Autodesk Inventor part; units mm, degrees
ref_plane "Work Plane1" through (0, 0, -15) normal (0, 0, 1) x (1, 0, 0)
ref_plane "YZ Plane" through (0, 0, 0) normal (1, 0, 0) x (0, 1, 0)
ref_plane "XZ Plane" through (0, 0, 0) normal (0, 1, 0) x (-1, 0, 0)
sketch "Sketch1" plane through (0, 0, 0) normal (0, 0, 1) x (1, 0, 0)
  line L0 (0, 0) -> (25, 0)
  line L1 (25, 0) -> (25, 40)
  line L2 (25, 40) -> (0, 40)
  line L3 (0, 40) -> (0, 0)
  dimension "d1" = 25
  dimension "d2" = 40
  dimension "d3" = 25
extrude "Extrusion1" add sketch "Sketch1" against normal blind 30
sketch "Sketch2" plane through (25, 0, 0) normal (1, 0, 0) x (0, 0, -1)
  line L0 (0, 0) -> (30, 0)
  circle A0 centre (15, 6.56) radius 2.46
extrude "Extrusion2" cut sketch "Sketch2" against normal blind 30
sketch "Sketch3" plane through (0, 0, 0) normal (-1, 0, 0) x (0, 0, 1)
  line L0 (0, 0) -> (-30, 0)
  line L1 (-25.05, 0) -> (-4.95, 0)
  line L2 (-4.95, 0) -> (-4.95, 33.12)
  line L3 (-4.95, 33.12) -> (-25.05, 33.12)
  line L4 (-25.05, 33.12) -> (-25.05, 0)
  dimension "d11" = 20.1
extrude "Extrusion3" cut sketch "Sketch3" against normal blind 20
sketch "Sketch4" plane through (0, 0, 0) normal (0, -1, 0) x (1, 0, 0)
  line L0 (20, -4.95) -> (20, -25.05)
  line L1 (20, -15) -> (25, -15)
  line L2 (25, 0) -> (25, -30)
  line L3 (20, -8.025) -> (25, -8.025)
  line L4 (25, -8.025) -> (25, -21.975)
  line L5 (25, -21.975) -> (20, -21.975)
  line L6 (20, -21.975) -> (20, -8.025)
  line L7 (20, -8.025) -> (25, -21.975) construction
  line L8 (25, -8.025) -> (20, -21.975) construction
  line L9 (25, -12.54) -> (25, -17.46)
  point P0 (0, 0)
  point P1 (22.5, -15)
  dimension "d14" = 13.95
extrude "Extrusion4" add sketch "Sketch4" along normal blind 15
sketch "Sketch5" plane through (20, 0, 0) normal (-1, 0, 0) x (0, 0, 1)
  circle A0 centre (-15, 6.56) radius 2.46
  circle A1 centre (-15, 6.56) radius 4.7025
  circle A2 centre (-15, 6.56) radius 2.46
  circle A3 centre (-15, 6.56) radius 2.46
  point P0 (0, 0)
  dimension "d17" = 9.405
extrude "Extrusion5" cut sketch "Sketch5" against normal blind 2.1
sketch "Sketch6" plane through (25, 0, 0) normal (1, 0, 0) x (0, 0, -1)
  circle A0 centre (15, 6.56) radius 4.7025
  line L0 (15, 6.56) -> (15, 23.56)
  circle A1 centre (15, 23.56) radius 2.46
  point P0 (0, 0)
  dimension "d20" = 17
  dimension "d21" = 4.92
extrude "Extrusion6" cut sketch "Sketch6" against normal blind 10 contours A1
sketch "Sketch7" plane through (20, 0, 0) normal (-1, 0, 0) x (0, 0, 1)
  circle A0 centre (-15, 23.56) radius 2.46
  circle A1 centre (-15, 23.56) radius 4.7025
  point P0 (0, 0)
  dimension "d24" = 9.405
extrude "Extrusion7" cut sketch "Sketch7" against normal blind 2.1
sketch "Sketch9" plane through (25, 0, 0) normal (1, 0, 0) x (0, 0, -1)
  circle A0 centre (15, 6.56) radius 2.46
  circle A1 centre (15, 6.56) radius 2.46
  circle A2 centre (15, 23.56) radius 2.46
  circle A3 centre (15, 23.56) radius 2.46
  line L0 (30, 40) -> (30, 0)
  line L1 (30, 0) -> (30, 40)
  line L2 (30, 40) -> (0, 40)
  line L3 (0, 40) -> (0, 0)
  line L4 (0, 0) -> (8.025, 0)
  line L5 (21.975, 0) -> (21.975, -15)
  line L6 (21.975, -15) -> (8.025, -15)
  line L7 (8.025, -15) -> (8.025, 0)
  line L8 (0, 0) -> (8.025, 0)
  line L9 (21.975, 0) -> (30, 0)
extrude "Extrusion8" add sketch "Sketch9" along normal blind 5
sketch "Sketch10" plane through (0, 40, 0) normal (0, 1, 0) x (1, 0, 0)
  line L0 (0, 30) -> (30, 30)
  line L1 (30, 0) -> (0, 0)
  line L2 (0, 30) -> (30, 30)
  line L3 (30, 30) -> (30, 0)
  line L4 (30, 0) -> (0, 0)
  line L5 (0, 0) -> (0, 30)
extrude "Extrusion9" add sketch "Sketch10" along normal blind 30
sketch "Sketch12" plane through (30, 0, 0) normal (1, 0, 0) x (0, 0, -1)
  circle A0 centre (15, 6.56) radius 2.46
  line L0 (15, 6.56) -> (15, 15.06)
  circle A1 centre (15, 15.06) radius 2.525
  point P0 (0, 0)
  dimension "d31" = 8.5
  dimension "d33" = 5.05
extrude "Extrusion10" cut sketch "Sketch12" against normal blind 30 contours A1
sketch "Sketch14" plane through (0, 0, 0) normal (0, 0, 1) x (1, 0, 0)
  line L0 (30, 70) -> (0, 70)
  line L1 (0, 100) -> (-8, 100)
  line L2 (30, 0) -> (30, 70)
  line L3 (30, 118) -> (30, 70)
  line L4 (30, 105) -> (30, 100)
  line L5 (0, 70) -> (30, 70)
  line L6 (0, 70) -> (0, 100)
  line L7 (30, 122.5) -> (30, 118)
  line L8 (-2, 150) -> (-8, 152)
  line L9 (-2, 102) -> (-8, 100)
  line L10 (-2, 102) -> (4, 126)
  line L11 (4, 126) -> (-2, 150)
  line L12 (-8, 152) -> (15, 152)
  line L13 (30, 137) -> (15, 152)
  line L14 (30, 122.5) -> (30, 137)
  point P0 (0, 0)
  dimension "d47" = 30
extrude "Extrusion12" add sketch "Sketch14" against normal blind 30
sketch "Sketch15" plane through (0, 0, -25.05) normal (-1, 0, 0) x (0, 0, 1)
  line L0 (0, 33.12) -> (20.1, 33.12)
  line L1 (20.1, 33.12) -> (20.1, 0)
  line L2 (0, 33.12) -> (20.1, 33.12)
  line L3 (20.1, 33.12) -> (20.1, 31.1)
  line L4 (20.1, 31.1) -> (0, 31.1)
  line L5 (0, 31.1) -> (0, 33.12)
  point P0 (25.05, 0)
  dimension "d57" = 2.02
extrude "Extrusion13" add sketch "Sketch15" against normal blind 20
sketch "Sketch25" plane through (0, 0, 0) normal (0, 0, 1) x (1, 0, 0)
  point P0 (0, 0)
sketch "Sketch26" plane through (0, 0, 0) normal (0, 0, 1) x (1, 0, 0)
  line L0 (-8, 100) -> (0, 100)
  line L1 (0, 100) -> (-8, 100)
  line L2 (-8, 100) -> (-2, 102)
  line L3 (-8, 100) -> (-2, 102)
  line L4 (-2, 102) -> (4, 126)
  line L5 (-2, 102) -> (4, 126)
  line L6 (4, 126) -> (-2, 150)
  line L7 (4, 126) -> (-2, 150)
  line L8 (-8, 152) -> (-2, 150)
  line L9 (-2, 150) -> (-8, 152)
  line L10 (15, 152) -> (-8, 152)
  line L11 (-8, 152) -> (15, 152)
  line L12 (30, 137) -> (15, 152)
  line L13 (15, 152) -> (30, 137)
  line L14 (30, 137) -> (30, 92)
  line L15 (30, 0) -> (30, 137)
  line L16 (30, 92) -> (0, 92)
  line L17 (0, 0) -> (0, 100)
  line L18 (0, 100) -> (0, 92)
  dimension "d93" = 45
extrude "Extrusion14" add sketch "Sketch26" along normal blind 45
ref_plane "Work Plane1" through (0, 0, -15) normal (0, 0, 1) x (1, 0, 0)
mirror "Mirror1" about plane through (0, 0, -15) normal (0, 0, 1) of "Extrusion14"
properties part number "48mm_x_120mm"
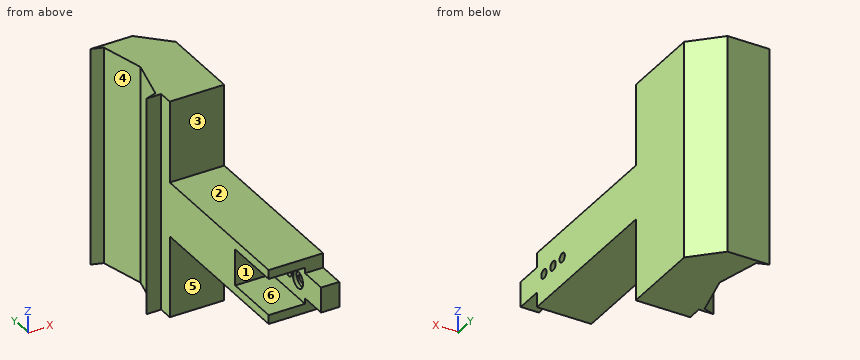
Geometry check sheet. Reference: the model listing, model coordinates, mm. Face numbers are marked on the shaded views. A direction names the side the tool comes from. Round coordinates to 2 decimals unless told otherwise and drop trailing zeros. Order: outer loops, then holes, each group sorted by start corner. A loop starts at its lowest first (then second) coordinate and runs counter-clockwise, first axis right, second up. Notation, with made-up numbers: (-1.75, 64) - (40.25, 64) arc R21 ccw to (40.25, 74) - close; hole circle Ø7 at (48.25, 84.25). An arc over 180 degrees is marked (long way). Use a Markdown table: item, result. Add a question column.
1) Thickness scan on line 1 along Z through (x, y) = (27.5, 23.56); line 2 along Z through (x, y) = (1.5, 25.5); line 3 along Y through (x, z) = (26.5, -15) (3 decimals). Record the ranges inside material, lowest first.
2) Section check A-A (z = -15). Count the separate pieces of the cut face and the enclosed holes in it, then the cut area to 3 significant figures.
3) Section check D-D (z = 24). Record the cut outline in (x, y), then the cut area to 3 significant figures.
4) Gauge pin test, flat ends, axial feed: P1, Ø9, axis at x = -6, z = -11, coming from the -Y side; P2, Ø12, axis at x = 2, z = -38.5, coming from the -Y side; P3, Ø4, axis at x = 22, z = -3, coming from the -Y side; P4, Ø3, axis at y = 6.56, z = -15, coming from the +X side. Record the tip position at first contact, or that the pin passes through.
5) Set-up check for the marked faces 4, 5 and 6: record each of +Z, -Z, +X, -X, +Y, -Y from which the full face is reachable in a straight line by a thin tool's end or side.
6) Section check C-C (y = 6.56). Record the cut outline in (x, z), then the cut area to 3 significant figures.
7) Section check B-B (x = 24). Record the cut outline in (y, z) (3 decimals), then the cut area to 3 significant figures.
8) Mould release check, pull along Z, two halves, no side actions. Record for the marked faces 1, 2 and 3: released by +Z, released by -Z, zero draft, split by the parting line, or undercut.
Established:
| question | item | result |
|---|---|---|
| 1 | line 1 | -30 to -17.46, -12.54 to 0 |
| 1 | line 2 | -30 to -25.05, -4.95 to 0 |
| 1 | line 3 | -15 to 4.1, 9.02 to 12.535, 17.585 to 21.1, 26.02 to 140.5 |
| 2 | separate pieces | 4 |
| 2 | enclosed holes | 0 |
| 2 | area | 3,780 mm2 |
| 3 | outline | (-8, 100) - (0, 100) - (0, 92) - (30, 92) - (30, 137) - (15, 152) - (-8, 152) - (-2, 150) - (4, 126) - (-2, 102) - close |
| 3 | area | 1,660 mm2 |
| 4 | P1 | y = 100 |
| 4 | P2 | y = 92 |
| 4 | P3 | y = 0 |
| 4 | P4 | through |
| 5 | face 4 | +Z, -Z, -X |
| 5 | face 5 | -Z, +X, -X, -Y |
| 5 | face 6 | -X, -Y |
| 6 | outline | (0, -30) - (30, -30) - (30, -17.46) - (22.1, -17.46) - (22.1, -19.7) - (20, -19.7) - (20, -25.05) - (0, -25.05) - close; (0, -4.95) - (20, -4.95) - (20, -10.3) - (22.1, -10.3) - (22.1, -12.54) - (30, -12.54) - (30, 0) - (0, 0) - close |
| 6 | area | 439 mm2 |
| 7 | outline | (-15, -21.975) - (0, -21.975) - (0, -30) - (92, -30) - (92, -75) - (143, -75) - (143, 45) - (92, 45) - (92, 0) - (0, 0) - (0, -8.025) - (-15, -8.025) - close; hole circle Ø4.92 at (6.56, -15); hole circle Ø5.05 at (15.06, -15); hole circle Ø4.92 at (23.56, -15) |
| 7 | area | 9,030 mm2 |
| 8 | face 1 | undercut |
| 8 | face 2 | released by +Z |
| 8 | face 3 | zero draft |
